from build123d import *

# Parameters (mm, degrees)
BOSS_EXTRUDE1_DEPTH = 9.525
FILLET1_R           = 1
FILLET2_R           = 2.54
SKETCH2_R           = 1.778
CUT_EXTRUDE1_DEPTH  = 26.295811414
SKETCH3_R           = 1.8288
CUT_EXTRUDE2_DEPTH  = 27.026870731


with BuildPart() as part:
    # Sketch1 → Boss-Extrude1 (new body)
    with BuildSketch(Plane.XY):
        Polygon((0, 0), (0, 20.6248), (12.7, 20.6248), (12.7, 19.05), (1.5748, 19.05), (1.5748, 0), align=None)
    extrude(amount=BOSS_EXTRUDE1_DEPTH)

    # Fillet1
    fillet1_edges = [part.edges().sort_by_distance(p)[0] for p in [
        (1.5748, 19.05, 4.7625),
    ]]
    fillet(fillet1_edges, radius=FILLET1_R)

    # Fillet2
    fillet2_edges = [part.edges().sort_by_distance(p)[0] for p in [
        (0, 20.6248, 4.7625),
    ]]
    fillet(fillet2_edges, radius=FILLET2_R)

    # Sketch2 → Cut-Extrude1 (cut, through all)
    with BuildSketch(Plane(origin=(1.5748, 0, 0), x_dir=(0, 0, -1), z_dir=(1, 0, 0))):
        with Locations(Location((-4.7625, 3.81, 0), (0, 0, 90))):
            Circle(SKETCH2_R)
    extrude(amount=-CUT_EXTRUDE1_DEPTH, mode=Mode.SUBTRACT)

    # Sketch3 → Cut-Extrude2 (cut, through all)
    with BuildSketch(Plane(origin=(0, 20.6248, 0), x_dir=(1, 0, 0), z_dir=(0, 1, 0))):
        with Locations(Location((7.3025, -4.7625, 0), (0, 0, 270))):
            Circle(SKETCH3_R)
    extrude(amount=-CUT_EXTRUDE2_DEPTH, mode=Mode.SUBTRACT)


solid = part.part
Geometry: final body of the model. Coordinates: model frame, mm. A direction names the side the tool comes from. Give positions to 0.01 mm unless a question says otherwise; leave off trailing zeros. Write each loop counter-clockwise with the first axis right and the second up, starting at its lowest first coordinate (ties: lowest second). Pieces come first, ordered by that corner, then holes.
(1) Cut plane B-B, the plane z = 2.25. Return loops of the section in (x, y), then the cut area to 3 significant figures.
(2) Cut plane A-A, the plane y = 3.81. Return loops of the section in (x, z) (1 decimal).
(3) Cut plane C-C, the plane z = 3.75. Return loops of the section in (x, y).
(4) Mould query, pull axis Y, two halves, no side actions, for faces 3 (the cylindrical face through (0.764, 19.9, 4.829)), 4 (the cylindrical face through (5.68, 19.85, 5.61)), 5 (the cylindrical face through (0.798, 3.425, 3.027)). Classes: released by +Y, released by -Y, zero draft, split by the parting line, or undercut.
(5) Ray query, line 1 (Z direction, x = 0.4, y = 3.81) (1 decimal); line 2 (Y direction, x = 3.25, z = 4.5); line 3 (X direction, y = 10.5, z = 8.25). Return the intervals inside material, ascending.
(6) Access query for faces 1 (the flat face through (0, 9, 5)), 2 (the flat face through (1.575, 9, 5)). Directions: +Z, -Z, +X, -X, +Y, -Y. A direction counts if a zero-diameter tool reaches every point of the face in a straight line with its end or side. Return the directions, or none.
(7) Cut plane D-D, the plane x = 3.75. Return loops of the section in (y, z) (3 decimals), then the cut area to 3 significant figures.
(8) First-contact query: P1, Ø3, axis at y = 10, z = 4, coming from the +X side; P2, Ø5, axis at x = 6, z = 2, coming from the -Y side; P3, Ø4, axis at x = 7.3, z = 4.76, coming from the +Y side; P4, Ø3, axis at y = 3.81, z = 4.76, coming from the +X side. Flat tips, straight axial feed; report the tip coordinate or a pass-through.
Values follow:
1. outline: (0, 0) - (1.57, 0) - (1.57, 18.05) arc R1 cw to (2.57, 19.05) - (12.7, 19.05) - (12.7, 20.62) - (2.54, 20.62) arc R2.54 ccw to (0, 18.08) - close
1. area: 48.8 mm2
2. outline: (0, 0) - (1.6, 0) - (1.6, 3) - (0, 3) - close; (0, 6.5) - (1.6, 6.5) - (1.6, 9.5) - (0, 9.5) - close
3. outline: (0, 0) - (1.57, 0) - (1.57, 2.35) - (0, 2.35) - close; (0, 5.27) - (1.57, 5.27) - (1.57, 18.05) arc R1 cw to (2.57, 19.05) - (5.78, 19.05) - (5.78, 20.62) - (2.54, 20.62) arc R2.54 ccw to (0, 18.08) - close; (8.83, 19.05) - (12.7, 19.05) - (12.7, 20.62) - (8.83, 20.62) - close
4. face 3: released by +Y
4. face 4: zero draft
4. face 5: undercut
5. line 1: z = 0 to 3, 6.5 to 9.5
5. line 2: y = 19.05 to 20.62
5. line 3: x = 0 to 1.57
6. face 1: +Z, -Z, -X, +Y, -Y
6. face 2: +Z, -Z, +X, -Y
7. outline: (19.05, 0) - (20.625, 0) - (20.625, 9.525) - (19.05, 9.525) - close
7. area: 15.0 mm2
8. P1: stops at x = 1.57
8. P2: stops at y = 19.05
8. P3: stops at y = 20.62
8. P4: passes through
